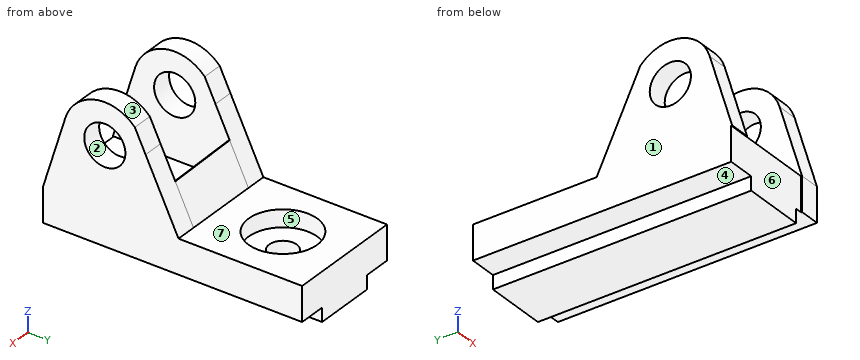
from build123d import *

# Parameters (mm, degrees)
SKETCH1_W            = 85
SKETCH1_H            = 90
SKETCH1_R            = 25
BOSS_EXTRUDE1_DEPTH  = 25
SKETCH1_3_R          = 25
SKETCH1_3_R_2        = 10
BOSS_EXTRUDE2_DEPTH  = 25
SKETCH1_5_R          = 10
CUT_EXTRUDE1_DEPTH   = 72.960881466
SKETCH1_6_R          = 25
SKETCH1_6_R_2        = 10
CUT_EXTRUDE2_DEPTH   = 12.5
SKETCH3_R            = 15
SKETCH3_W            = 25
SKETCH3_H            = 98.657332742
BOSS_EXTRUDE3_DEPTH  = 15
SKETCH5_W            = 25
SKETCH5_H            = 98.657332742
CUT_EXTRUDE3_DEPTH   = 15
SKETCH8_W            = 85
SKETCH8_H            = 25
BOSS_EXTRUDE8_DEPTH  = 98
BOSS_EXTRUDE9_DEPTH  = 1
SKETCH12_W           = 45
SKETCH12_H           = 10
BOSS_EXTRUDE11_DEPTH = 188
CUT_EXTRUDE4_DEPTH   = 177.647203174


with BuildPart() as part:
    # Sketch1 → Boss-Extrude1 (new body)
    with BuildSketch(Plane.XY):
        with Locations((-7.652354571, -0.145429363)):
            Rectangle(SKETCH1_W, SKETCH1_H)
        with Locations((-7.652354571, 0)):
            Circle(SKETCH1_R, mode=Mode.SUBTRACT)
    extrude(amount=-BOSS_EXTRUDE1_DEPTH)

    # Sketch3 → Boss-Extrude3 (add)
    # profile 1 of 2: a face of its own
    with BuildSketch(Plane(origin=(34.847645429, 0, 0), x_dir=(0, 0, -1), z_dir=(1, 0, 0))):
        with BuildLine():
            Line((0, -143.802762105), (0, -45.145429363))
            Line((0, -45.145429363), (-49.456840406, -69.135666299))
            Line((-49.456840406, -69.135666299), (-65.54026385, -76.937319943))
            ThreePointArc((-65.54026385, -76.937319943), (-74.211212735, -105.636871453), (-53.708286934, -127.511049039))
            Line((-53.708286934, -127.511049039), (0, -143.802762105))
        make_face()
        with Locations(Location((-45, -98.802762105, 0), (0, 0, 90))):
            Circle(SKETCH3_R, mode=Mode.SUBTRACT)
    # profile 2 of 2: a face of its own
    with BuildSketch(Plane(origin=(34.847645429, 0, 0), x_dir=(0, 0, -1), z_dir=(1, 0, 0))):
        with Locations((12.5, -94.474095734)):
            Rectangle(SKETCH3_W, SKETCH3_H)
    extrude(amount=-BOSS_EXTRUDE3_DEPTH)


with BuildPart() as body_2:
    # Sketch1<3> → Boss-Extrude2 (new body)
    # profile 1 of 2: a face of its own
    with BuildSketch(Plane.XY):
        with Locations((-7.652354571, 0)):
            Circle(SKETCH1_3_R)
        with Locations((-7.652354571, 0)):
            Circle(SKETCH1_3_R_2, mode=Mode.SUBTRACT)
    # profile 2 of 2: a face of its own
    with BuildSketch(Plane.XY):
        with Locations((-7.652354571, 0)):
            Circle(SKETCH1_3_R_2)
    extrude(amount=-BOSS_EXTRUDE2_DEPTH)

    # Sketch1<5> → Cut-Extrude1 (cut, through all)
    with BuildSketch(Plane.XY):
        with Locations((-7.652354571, 0)):
            Circle(SKETCH1_5_R)
    extrude(amount=-CUT_EXTRUDE1_DEPTH, mode=Mode.SUBTRACT)

    # Sketch1<6> → Cut-Extrude2 (cut)
    with BuildSketch(Plane.XY):
        with Locations((-7.652354571, 0)):
            Circle(SKETCH1_6_R)
        with Locations((-7.652354571, 0)):
            Circle(SKETCH1_6_R_2, mode=Mode.SUBTRACT)
    extrude(amount=-CUT_EXTRUDE2_DEPTH, mode=Mode.SUBTRACT)


with BuildPart() as body_3:
    # Mirror1: mirrored copy
    add(part.part.mirror(Plane(origin=(-7.652354571, 0, 0), x_dir=(0, 0, 1), z_dir=(1, 0, 0))))

    # Sketch5 → Cut-Extrude3 (cut)
    with BuildSketch(Plane.ZY.offset(50.152354571)):
        with Locations((-12.5, -94.474095734)):
            Rectangle(SKETCH5_W, SKETCH5_H)
    extrude(amount=-CUT_EXTRUDE3_DEPTH, mode=Mode.SUBTRACT)


with BuildPart() as cut_extrude3_piece_1:
    # of the separate pieces the step leaves, piece 1, a body of its own (cut_extrude3_pieces)
    add(body_3.part.solids().sort_by_distance((34.847645429, -45.145429363, 0))[0])


with BuildPart() as cut_extrude3_piece_2:
    # of the separate pieces the step leaves, piece 2, a body of its own (cut_extrude3_pieces)
    add(body_3.part.solids().sort_by_distance((-35.152354571, -76.937319943, 65.54026385))[0])


with BuildPart() as part_1:
    add(part.part)

    add(cut_extrude3_piece_1.part)  # Boss-Extrude8 merges Cut-Extrude3 piece 1

    add(cut_extrude3_piece_2.part)  # Boss-Extrude8 merges Cut-Extrude3 piece 2
    # Sketch8 → Boss-Extrude8 (add)
    with BuildSketch(Plane.XZ.offset(45.145429363)):
        with Locations((-7.652354571, -12.5)):
            Rectangle(SKETCH8_W, SKETCH8_H)
    extrude(amount=BOSS_EXTRUDE8_DEPTH)

    # Sketch9 → Boss-Extrude9 (add)
    with BuildSketch(Plane(origin=(0, -36.5462155, -17.727625982), x_dir=(1, 0, 0), z_dir=(0, 0.8997343711779642, 0.4364379237887027))):
        Polygon((-50.152354571, -51.174548766), (34.847645429, -49.760817749), (34.847645429, -19.70317746), (-50.152354571, -19.70317746), align=None)
    extrude(amount=-BOSS_EXTRUDE9_DEPTH)

    add(body_2.part)  # Boss-Extrude11 merges body 2
    # Sketch12 → Boss-Extrude11 (add)
    with BuildSketch(Plane(origin=(0, 44.854570637, 0), x_dir=(1, 0, 0), z_dir=(0, 1, 0))):
        with Locations((-7.652354571, 30)):
            Rectangle(SKETCH12_W, SKETCH12_H)
    extrude(amount=-BOSS_EXTRUDE11_DEPTH)

    # Sketch11 → Cut-Extrude4 (cut, through all)
    with BuildSketch(Plane(origin=(19.847645429, 0, 0), x_dir=(0, 0, -1), z_dir=(1, 0, 0))):
        Polygon((0, -143.802762105), (-26.854143467, -135.656905572), (-27, -143.802762105), align=None)
    extrude(amount=-CUT_EXTRUDE4_DEPTH, mode=Mode.SUBTRACT)


solid = part_1.part
Could you check a few things on this model? Use its own coordinates, in mm. Face numbers are marked on the shaded views. A direction names the side the tool comes from. Give positions to 0.01 mm unless a question says otherwise; leave off trailing zeros. Loops run counter-clockwise (first coordinate to the right, second up) from the corner with the lowest first, then second, coordinate; pieces in that order, holes last. Notation, with made-up numbers: M 48.25,-35 L 94.25,-35 A3 ccw 94.25,-30 Z; hole C -5,88.5 d9. An arc over 180 degrees is marked long. Answer as a JSON object with one key per item and string values.
Q1. Suppose I cut it at D-D, the plane x = 9.5. List the corners of the cut face in (y, z) for me, plus the area to 3 significant figures.
Values found:
{"outline": "M -143.15,-35 L 44.85,-35 L 44.85,0 L 18.19,0 L 18.19,-12.5 L -18.19,-12.5 L -18.19,0 L -45.15,0 L -58.45,27.42 L -59.35,26.99 L -46.26,0 L -143.15,0 Z", "area": "6,160 mm²"}
Q2. If I drill on probe 1 along X at (y, z) = (0, -5); probe 2 along X at (y, z) = (-111, 33); probe 3 along Y at (x, z) = (-39, -15.5), over which ranges is the centre line in solid material (lowest first)? Write a range as [from, to].
Values found:
{"probe 1": "x = [-50.15, -32.65], [17.35, 34.85]", "probe 2": "x = [-50.15, -35.15], [19.85, 34.85]", "probe 3": "y = [-143.15, 44.85]"}
Q3. Suppose I cut it at C-C, the plane z = 45. List the corners of the cut face in (x, y) for me.
Values found:
{"outline": "M -50.15,-130.15 L -35.15,-130.15 L -35.15,-113.8 L -50.15,-113.8 Z; M -50.15,-83.8 L -35.15,-83.8 L -35.15,-66.97 L -50.15,-66.97 Z; M 19.85,-130.15 L 34.85,-130.15 L 34.85,-113.8 L 19.85,-113.8 Z; M 19.85,-83.8 L 34.85,-83.8 L 34.85,-66.97 L 19.85,-66.97 Z"}
Q4. Suppose I cut it at B-B, the plane y = -91. List the corners of the cut face in (x, z) for me.
Values found:
{"outline": "M -50.15,-25 L -30.15,-25 L -30.15,-35 L 14.85,-35 L 14.85,-25 L 34.85,-25 L 34.85,32.19 L 19.85,32.19 L 19.85,0 L -35.15,0 L -35.15,32.19 L -50.15,32.19 Z; M -50.15,57.81 L -35.15,57.81 L -35.15,73.97 L -50.15,73.97 Z; M 19.85,57.81 L 34.85,57.81 L 34.85,73.97 L 19.85,73.97 Z"}
Q5. For the marked faces 4, 5, 6 and 7, which set-ups out of +Z, -Z, +X, -X, +Y, -Y let a thin tool reach every point of the face, with its end or its side?
Values found:
{"face 4": "-Z, -X, +Y, -Y", "face 5": "+Z", "face 6": "-Z, -X, -Y", "face 7": "+Z, +X, -X, +Y"}
Q6. Suppose I cut it at A-A, the plane y = 0. List the corners of the cut face in (x, z) for me.
Values found:
{"outline": "M -50.15,-25 L -30.15,-25 L -30.15,-35 L 14.85,-35 L 14.85,-25 L 34.85,-25 L 34.85,0 L 17.35,0 L 17.35,-12.5 L 2.35,-12.5 L 2.35,-25 L -17.65,-25 L -17.65,-12.5 L -32.65,-12.5 L -32.65,0 L -50.15,0 Z"}
Q7. If we mould it in two halves opening along Z, with no side actions, what happens to the marked faces 1, 2 and 3? For each: pulls with the +Z half, pulls with the -Z half, needs draft (parallel to the pull), parting line crosses it, or undercut.
Values found:
{"face 1": "needs draft", "face 2": "undercut", "face 3": "pulls with the +Z half"}
Q8. For P1, Ø22, axis at x = -38.5, y = -31, coming from the -Z side; P2, Ø1, axis at x = -37, y = -52.5, coming from the +Z side; P3, Ø17.5, axis at x = -27.5, z = -22.5, coming from the -Y side; P4, Ø2, axis at x = -7.5, y = -114.5, coming from the +Z side, each with a flat end and sliding along its axis, tell me the tip position at first contact or that it passes through.
Values found:
{"P1": "stops at z = -35", "P2": "stops at z = 16.19", "P3": "stops at y = -143.15", "P4": "stops at z = 0"}
